Verification items for the finished model (mm, model axes). A direction names the side the tool comes from. Round coordinates to 2 decimals unless told otherwise and drop trailing zeros. Write each loop counter-clockwise with the first axis right and the second up, starting at its lowest first coordinate (ties: lowest second). Pieces come first, ordered by that corner, then holes. Notation, with made-up numbers: (56.5, -3.75) - (107.5, -3.75) arc R16 cw to (107.5, 24.25) - close; hole circle Ø3 at (40.5, -4.75). An arc over 180 degrees is marked (long way). Answer as a JSON object with one key per item and string values.
```python
from build123d import *

# Parameters (mm, degrees)
SKETCH_1_R          = 8.75
SKETCH_1_R_2        = 8.25
EXTRUDE_2_DEPTH     = 10
SKETCH_2_R          = 8.25
SKETCH_2_R_2        = 2
EXTRUDE_3_DEPTH     = 4
EXTRUDE_4_DEPTH     = 8
SKETCH_5_W          = 3
SKETCH_5_H          = 8
EXTRUDE_5_DEPTH     = 3
SKETCH_6_W          = 3
SKETCH_6_H          = 8
EXTRUDE_6_DEPTH     = 3
SKETCH_7_R          = 1.5
CUT_EXTRUDE_1_DEPTH = 3
FILLET_1_R          = 5
FILLET_3_R          = 2
SKETCH_8_R          = 8.75
SKETCH_8_R_2        = 8.25
EXTRUDE_7_DEPTH     = 8
SKETCH_9_R          = 8.25
SKETCH_9_R_2        = 6
EXTRUDE_8_DEPTH     = 2
EXTRUDE_9_DEPTH     = 8
SKETCH_11_R         = 1.5
CUT_EXTRUDE_2_DEPTH = 8
CUT_EXTRUDE_3_DEPTH = 8
CUT_EXTRUDE_4_DEPTH = 8
SKETCH_14_R         = 8.75
SKETCH_14_R_2       = 8.25
EXTRUDE_10_DEPTH    = 8
EXTRUDE_11_DEPTH    = 8
SKETCH_16_R         = 1.5
CUT_EXTRUDE_5_DEPTH = 8
CUT_EXTRUDE_6_DEPTH = 10


with BuildPart() as part:
    # 草图1 → 凸台-拉伸2 (new body)
    with BuildSketch(Plane(origin=(0, 0, 0), x_dir=(1, 0, 0), z_dir=(0, 1, 0))):
        Circle(SKETCH_1_R)
        Circle(SKETCH_1_R_2, mode=Mode.SUBTRACT)
    extrude(amount=EXTRUDE_2_DEPTH)

    # 草图2 → 凸台-拉伸3 (add)
    with BuildSketch(Plane(origin=(0, 0, 0), x_dir=(1, 0, 0), z_dir=(0, 1, 0))):
        Circle(SKETCH_2_R)
        Circle(SKETCH_2_R_2, mode=Mode.SUBTRACT)
    extrude(amount=EXTRUDE_3_DEPTH)

    # 草图3 → 凸台-拉伸4 (add)
    with BuildSketch(Plane(origin=(0, 0, 0), x_dir=(1, 0, 0), z_dir=(0, 1, 0))):
        Polygon((-2, 8.518362519), (2, 8.518362519), (2, 15), (15, 15), (15, 18), (2, 18), (-2, 18), (-15, 18), (-15, 15), (-2, 15), align=None)
    extrude(amount=EXTRUDE_4_DEPTH)

    # 草图5 → 凸台-拉伸5 (add)
    with BuildSketch(Plane(origin=(15, 0, 0), x_dir=(0, 0, -1), z_dir=(1, 0, 0))):
        with Locations((16.5, 4)):
            Rectangle(SKETCH_5_W, SKETCH_5_H)
    extrude(amount=EXTRUDE_5_DEPTH)

    # 草图6 → 凸台-拉伸6 (add)
    with BuildSketch(Plane.ZY.offset(15)):
        with Locations((-16.5, 4)):
            Rectangle(SKETCH_6_W, SKETCH_6_H)
    extrude(amount=EXTRUDE_6_DEPTH)

    # 草图7 → 切除-拉伸1 (cut)
    with BuildSketch(Plane(origin=(0, 0, -18), x_dir=(-1, 0, 0), z_dir=(0, 0, -1))):
        with Locations((-15, 3.754021035)):
            Circle(SKETCH_7_R)
    cut_extrude_1 = extrude(amount=-CUT_EXTRUDE_1_DEPTH, mode=Mode.SUBTRACT)

    # 镜向1: 切除-拉伸1 across plane
    add(cut_extrude_1.mirror(Plane(origin=(0, 0, 0), x_dir=(0, 0, 1), z_dir=(1, 0, 0))), mode=Mode.SUBTRACT)

    # 圆角1
    fillet_1_edges = [part.edges().sort_by_distance(p)[0] for p in [
        (-2, 4, -8.518362519),
        (2, 4, -8.518362519),
    ]]
    fillet(fillet_1_edges, radius=FILLET_1_R)

    # 圆角3
    fillet_3_edges = [part.edges().sort_by_distance(p)[0] for p in [
        (-2, 4, -15),
        (2, 4, -15),
    ]]
    fillet(fillet_3_edges, radius=FILLET_3_R)


with BuildPart() as body_2:
    # 草图8 → 凸台-拉伸7 (new body)
    with BuildSketch(Plane(origin=(0, 0, 0), x_dir=(1, 0, 0), z_dir=(0, 1, 0))):
        with Locations((27.184954533, 0)):
            Circle(SKETCH_8_R)
        with Locations((27.184954533, 0)):
            Circle(SKETCH_8_R_2, mode=Mode.SUBTRACT)
    extrude(amount=EXTRUDE_7_DEPTH)

    # 草图9 → 凸台-拉伸8 (add)
    with BuildSketch(Plane.XZ):
        with Locations((27.184954533, 0)):
            Circle(SKETCH_9_R)
        with Locations((27.184954533, 0)):
            Circle(SKETCH_9_R_2, mode=Mode.SUBTRACT)
    extrude(amount=-EXTRUDE_8_DEPTH)

    # 草图10 → 凸台-拉伸9 (add)
    with BuildSketch(Plane(origin=(0, 0, 0), x_dir=(1, 0, 0), z_dir=(0, 1, 0))):
        Polygon((27.184954533, -18), (45.184954533, -18), (45.184954533, -14.663867829), (29.184954533, -14.663867829), (29.184954533, -8.518362519), (25.184954533, -8.518362519), (25.184954533, -14.663867829), (9.184954533, -14.663867829), (9.184954533, -18), align=None)
    extrude(amount=EXTRUDE_9_DEPTH)

    # 草图11 → 切除-拉伸2 (cut)
    with BuildSketch(Plane.XY.offset(18)):
        with Locations((12.184954533, 4)):
            Circle(SKETCH_11_R)
        with Locations((42.184954533, 4)):
            Circle(SKETCH_11_R)
    extrude(amount=-CUT_EXTRUDE_2_DEPTH, mode=Mode.SUBTRACT)

    # 草图12 → 切除-拉伸3 (cut)
    with BuildSketch(Plane.XY.offset(18)):
        with BuildLine():
            Line((10.684954533, 4), (10.684954533, 5))
            ThreePointArc((10.684954533, 5), (12.184954533, 6.5), (13.684954533, 5))
            Line((13.684954533, 5), (13.684954533, 4))
            Line((13.684954533, 4), (13.684954533, 3))
            ThreePointArc((13.684954533, 3), (12.184954533, 1.5), (10.684954533, 3))
            Line((10.684954533, 3), (10.684954533, 4))
        make_face()
    extrude(amount=-CUT_EXTRUDE_3_DEPTH, mode=Mode.SUBTRACT)

    # 草图13 → 切除-拉伸4 (cut)
    with BuildSketch(Plane.XY.offset(18)):
        with BuildLine():
            Line((40.684954533, 4), (40.684954533, 5))
            ThreePointArc((40.684954533, 5), (42.184954533, 6.5), (43.684954533, 5))
            Line((43.684954533, 5), (43.684954533, 4))
            Line((43.684954533, 4), (43.684954533, 3))
            ThreePointArc((43.684954533, 3), (42.184954533, 1.5), (40.684954533, 3))
            Line((40.684954533, 3), (40.684954533, 4))
        make_face()
    extrude(amount=-CUT_EXTRUDE_4_DEPTH, mode=Mode.SUBTRACT)


with BuildPart() as body_3:
    # 草图14 → 凸台-拉伸10 (new body)
    with BuildSketch(Plane(origin=(0, 0, 0), x_dir=(1, 0, 0), z_dir=(0, 1, 0))):
        with Locations((-35.091635024, 0)):
            Circle(SKETCH_14_R)
        with Locations((-35.091635024, 0)):
            Circle(SKETCH_14_R_2, mode=Mode.SUBTRACT)
    extrude(amount=EXTRUDE_10_DEPTH)

    # 草图15 → 凸台-拉伸11 (add)
    with BuildSketch(Plane(origin=(0, 0, 0), x_dir=(1, 0, 0), z_dir=(0, 1, 0))):
        Polygon((-37.091635024, -15), (-37.091635024, -8.518362519), (-33.091635024, -8.518362519), (-33.091635024, -15), (-17.091635024, -15), (-17.091635024, -18), (-53.091635024, -18), (-53.091635024, -15), align=None)
    extrude(amount=EXTRUDE_11_DEPTH)

    # 草图16 → 切除-拉伸5 (cut)
    with BuildSketch(Plane.XY.offset(18)):
        with Locations((-50.091635024, 4)):
            Circle(SKETCH_16_R)
        with Locations((-20.091635024, 4)):
            Circle(SKETCH_16_R)
    extrude(amount=-CUT_EXTRUDE_5_DEPTH, mode=Mode.SUBTRACT)


with BuildPart() as cut_extrude_6_tool:
    # 草图17 → 切除-拉伸6 (new body)
    with BuildSketch(Plane(origin=(0, 0, 0), x_dir=(1, 0, 0), z_dir=(0, 1, 0))):
        Polygon((-22.814109192, 34.802391794), (-16.193349778, -3.968895549), (-7.026713263, -18.825168522), (52.714469541, -30.836623265), (64.093742456, -10), (34.287483401, 32.08598291), align=None)
    extrude(amount=CUT_EXTRUDE_6_DEPTH)


with BuildPart() as part_1:
    add(part.part)

    # 切除-拉伸6: cut by cut_extrude_6_tool
    add(cut_extrude_6_tool.part, mode=Mode.SUBTRACT)


with BuildPart() as body_2_1:
    add(body_2.part)

    # 切除-拉伸6: cut by cut_extrude_6_tool
    add(cut_extrude_6_tool.part, mode=Mode.SUBTRACT)


solid = body_3.part
```
1. Material ranges on probe 1 along Z at (x, y) = (-37.5, 3); probe 2 along Z at (x, y) = (-21, 0.5); probe 3 along Z at (x, y) = (-41, 6.25), recorded low to high. Write a range as from..to.
Completed:
{"probe 1": "z = -8.41..-7.89, 7.89..8.41, 15..18", "probe 2": "z = 15..18", "probe 3": "z = -6.45..-5.76, 5.76..6.45, 15..18"}
2. Go/stop test with flat-tipped pins: pin 1 (3.5 mm diameter, centred on x = -20.09, y = 4, fed in from +Z); pin 2 (3 mm diameter, centred on y = 6, z = 12, fed in from +X); pin 3 (1.9 mm diameter, centred on y = 4, z = 12.5, fed in from -X); pin 4 (2 mm diameter, centred on x = -40, y = 1, fed in from -Z). Record where each tip stops, or that it passes through.
Completed:
{"pin 1": "stops at z = 18", "pin 2": "stops at x = -33.09", "pin 3": "stops at x = -37.09", "pin 4": "stops at z = -7.83"}
3. Access from +Z, -Z, +X, -X, +Y, -Y to the whole of each face (thin tool, end or side, straight path). Record for faces 1 (the face through (-43.334, 3.944, -0.363)), 2 (the face through (-33.092, 4, 12)), 3 (the face through (-37.092, 4, 12)).
Completed:
{"face 1": "+Y, -Y", "face 2": "+X, +Y, -Y", "face 3": "-X, +Y, -Y"}
4. Cross-section at C-C (y = 1.5). Record the boundary of the cut face in (x, z), plus the area to 3 significant figures.
Completed:
{"outline": "(-53.09, 15) - (-37.09, 15) - (-37.09, 8.52) arc R8.75 ccw (long way) to (-33.09, 8.52) - (-33.09, 15) - (-17.09, 15) - (-17.09, 18) - (-53.09, 18) - close; hole circle Ø16.5 at (-35.09, 0)", "area": "160 mm^2"}
5. Cross-section at B-B (z = 0). Record the boundary of the cut face in (x, y), plus the area to 3 significant figures.
Completed:
{"outline": "(-43.84, 0) - (-43.34, 0) - (-43.34, 8) - (-43.84, 8) - close; (-26.84, 0) - (-26.34, 0) - (-26.34, 8) - (-26.84, 8) - close", "area": "8.00 mm^2"}
6. Cross-section at D-D (x = -34). Record the boundary of the cut face in (y, z), plus the area to 3 significant figures.
Completed:
{"outline": "(0, -8.68) - (8, -8.68) - (8, -8.18) - (0, -8.18) - close; (0, 8.18) - (8, 8.18) - (8, 18) - (0, 18) - close", "area": "82.6 mm^2"}
7. Mould release check, pull along Y, two halves, no side actions. Record for faces 4 (the face through (-51.282, 3.087, 16.521)), 5 (the face through (-21.59, 4.07, 16.52)), 6 (the face through (-45, 4, 15)), 7 (the face through (-35, 8, 12)): released by +Y, released by -Y, zero draft, split by the parting line, or undercut.
Completed:
{"face 4": "undercut", "face 5": "undercut", "face 6": "zero draft", "face 7": "released by +Y"}
8. Cross-section at A-A (y = 4). Record the boundary of the cut face in (x, z).
Completed:
{"outline": "(-53.09, 15) - (-51.59, 15) - (-51.59, 18) - (-53.09, 18) - close; (-48.59, 15) - (-37.09, 15) - (-37.09, 8.52) arc R8.75 ccw (long way) to (-33.09, 8.52) - (-33.09, 15) - (-21.59, 15) - (-21.59, 18) - (-48.59, 18) - close; (-18.59, 15) - (-17.09, 15) - (-17.09, 18) - (-18.59, 18) - close; hole circle Ø16.5 at (-35.09, 0)"}
